The listing builds one solid part. Answer for the finished solid, in the listing's coordinates (mm). Coordinates: 2 decimals unless noted, no trailing zeros. Order: outer loops, then holes, each group sorted by start corner. A loop starts at its lowest first (then second) coordinate and runs counter-clockwise, first axis right, second up. Notation, with made-up numbers: (-4.75, 65) -> (21.25, 65) arc R21 ccw to (21.25, 103) -> close; hole circle Ø9 at (-29, 73). An arc over 180 degrees is marked (long way). Return JSON: item names as keys, results as strings.
from build123d import *

# Parameters (mm, degrees)
SKETCH1_R           = 1.75
SKETCH1_R_2         = 2.3625
BOSS_EXTRUDE1_DEPTH = 2
SKETCH1_2_R         = 2.3625
BOSS_EXTRUDE2_DEPTH = 16.5


with BuildPart() as part:
    # Sketch1 → Boss-Extrude1 (new body)
    with BuildSketch(Plane.XY):
        Polygon((-9.5, -8), (-9.5, 8), (-4.688228281, 8), (4.5, 2.566962921), (4.5, -2.566962921), (-4.688228281, -8), align=None)
        with Locations((-6, -5)):
            Circle(SKETCH1_R, mode=Mode.SUBTRACT)
        with Locations((-6, 5)):
            Circle(SKETCH1_R, mode=Mode.SUBTRACT)
        Circle(SKETCH1_R_2, mode=Mode.SUBTRACT)
    extrude(amount=BOSS_EXTRUDE1_DEPTH)

    # Sketch1<2> → Boss-Extrude2 (add)
    with BuildSketch(Plane.XY):
        Circle(SKETCH1_2_R)
    extrude(amount=BOSS_EXTRUDE2_DEPTH)


solid = part.part
1. The part is cut by section A-A on z = 1.5. Give the vertices of the cut face in (x, y).
Answer block:
{"outline": "(-9.5, -8) -> (-4.69, -8) -> (4.5, -2.57) -> (4.5, 2.57) -> (-4.69, 8) -> (-9.5, 8) -> close; hole circle Ø3.5 at (-6, -5); hole circle Ø3.5 at (-6, 5)"}
2. Determine the mould class of faces 1 (the face through (2.253, 0.71, 9.148)), 2 (the face through (-4, 0, 2)), 3 (the face through (-6.38, 3.29, 0.99)) for opening direction Y: pulls with the +Y half, pulls with the -Y half, needs draft (parallel to the pull), parting line crosses it, or undercut.
Answer block:
{"face 1": "parting line crosses it", "face 2": "needs draft", "face 3": "undercut"}
3. Consider line 1 (Y direction, x = -6, z = 1.6); line 2 (Z direction, x = -5.25, y = 1); line 3 (Y direction, x = 1.5, z = 8). Determine where each line is inside the solid, lowest interval first. Write a range as from..to.
Answer block:
{"line 1": "y = -8..-6.75, -3.25..3.25, 6.75..8", "line 2": "z = 0..2", "line 3": "y = -1.83..1.83"}
4. Each of these flat-tipped pins is pushed along its axis until it touches: pin 1 Ø2 at (x, y) = (-3, -4) entering from +Z; pin 2 Ø8 at (y, z) = (-2.5, 10) entering from +X; pin 3 Ø3 at (x, z) = (2.5, 5) entering from -Y. Where does it stop, or does it pass through?
Answer block:
{"pin 1": "stops at z = 2", "pin 2": "stops at x = 2.36", "pin 3": "stops at y = -2.14"}
5. The part is cut by section C-C on y = -5. Give the vertices of the cut face in (x, z).
Answer block:
{"outline": "(-9.5, 0) -> (-7.75, 0) -> (-7.75, 2) -> (-9.5, 2) -> close; (-4.25, 0) -> (0.39, 0) -> (0.39, 2) -> (-4.25, 2) -> close"}
6. The part is cut by section B-B on x = -6. Give the vertices of the cut face in (y, z).
Answer block:
{"outline": "(-8, 0) -> (-6.75, 0) -> (-6.75, 2) -> (-8, 2) -> close; (-3.25, 0) -> (3.25, 0) -> (3.25, 2) -> (-3.25, 2) -> close; (6.75, 0) -> (8, 0) -> (8, 2) -> (6.75, 2) -> close"}
7. The part is cut by section D-D on y = 0. Give the vertices of the cut face in (x, z), and give its area (3 significant figures).
Answer block:
{"outline": "(-9.5, 0) -> (4.5, 0) -> (4.5, 2) -> (2.36, 2) -> (2.36, 16.5) -> (-2.36, 16.5) -> (-2.36, 2) -> (-9.5, 2) -> close", "area": "96.5 mm2"}
